Build history of the part. All positions in model axes, mm. A direction names the side the tool comes from. Give positions to 0.01 mm unless a question says otherwise; leave off trailing zeros. Loops run counter-clockwise (first coordinate to the right, second up) from the corner with the lowest first, then second, coordinate; pieces in that order, holes last. Notation, with made-up numbers: (64, 14) - (120, 14) arc R21 ccw to (120, 31) - close; hole circle Ø5 at (-3.75, 39.5). An arc over 180 degrees is marked (long way). Return JSON: item names as keys, results as strings. Group by question number.
1) Slice it at D-D (z = 1.25). List the corners of the cut face in (x, y).
2) Mould opens along X. For faces 1 (the face through (-53, -22, 3.48)), 2 (the face through (-45, -22, 3.48)), 3 (the face through (-50, -19, 0)), 4 (the face through (-41.453, -22, 2)) say: released by +X, released by -X, zero draft, split by the parting line, or undercut.
3) Slice it at A-A (z = 3). List the corners of the cut face in (x, y), and give its area (3 significant figures).
4) Drop a flat-ended pin along its axis: pin 1 (1.5 mm diameter, centred on x = -46, y = -22, fed in from -Z). Give the stop position or say it passes through.
5) Slice it at B-B (z = 4.3). List the corners of the cut face in (x, y), and give its area (3 significant figures).
6) Slice it at C-C (y = -20.25). List the corners of the cut face in (x, z) (3 decimals), and give its area (3 significant figures).
7) 3-axis set-ups, long thin cutter, end or side, ignore diameter. For faces 5 (the face through (-50, -25.879, 2)), 6 (the face through (-50, -22, 3.175)), 7 (the face through (-49, -24.279, 1)): which of +Z, -Z, +X, -X, +Y, -Y reach the whole face in a straight line?
8) Drill centre lines: probe 1 along X at (y, z) = (-23.5, 0.5); probe 2 along Y at (x, z) = (-49.5, 0.7); probe 3 along Z at (x, y) = (-53, -22.25). Where is each one in solid material? Low to high. Write a range as from..to.
```python
from build123d import *

# Parameters (mm, degrees)
F1_DEPTH = 3.175
F2_DEPTH = 5.08
F3_T     = -1.6002


with BuildPart() as f1:
    # F0 (on Top) → F1 (new body)
    with BuildSketch(Plane.XY):
        with BuildLine():
            Line((-53.3784843279, -17.9285755823), (-57.3535843279, -17.9285755823))
            Line((-57.3535843279, -17.9285755823), (-57.3535843279, -25.8787755823))
            Line((-57.3535843279, -25.8787755823), (-53.3784843279, -25.8787755823))
            Line((-53.3784843279, -25.8787755823), (-53.3784843279, -24.4436755823))
            ThreePointArc((-53.3784843279, -24.4436755823), (-55.9184843279, -21.9036755823), (-53.3784843279, -19.3636755823))
            Line((-53.3784843279, -19.3636755823), (-53.3784843279, -17.9285755823))
        make_face()
        with BuildLine():
            Line((-45.4282843279, -17.9285755823), (-53.3784843279, -17.9285755823))
            Line((-53.3784843279, -17.9285755823), (-53.3784843279, -19.3636755823))
            ThreePointArc((-53.3784843279, -19.3636755823), (-51.5824331037, -20.1076243581), (-50.8384843279, -21.9036755823))
            ThreePointArc((-50.8384843279, -21.9036755823), (-51.5824331037, -23.6997268065), (-53.3784843279, -24.4436755823))
            Line((-53.3784843279, -24.4436755823), (-53.3784843279, -25.8787755823))
            Line((-53.3784843279, -25.8787755823), (-45.4282843279, -25.8787755823))
            Line((-45.4282843279, -25.8787755823), (-45.4282843279, -24.4436755823))
            ThreePointArc((-45.4282843279, -24.4436755823), (-47.9682843279, -21.9036755823), (-45.4282843279, -19.3636755823))
            Line((-45.4282843279, -19.3636755823), (-45.4282843279, -17.9285755823))
        make_face()
        with BuildLine():
            Line((-41.4531843279, -17.9285755823), (-45.4282843279, -17.9285755823))
            Line((-45.4282843279, -17.9285755823), (-45.4282843279, -19.3636755823))
            ThreePointArc((-45.4282843279, -19.3636755823), (-43.6322331037, -20.1076243581), (-42.8882843279, -21.9036755823))
            ThreePointArc((-42.8882843279, -21.9036755823), (-43.6322331037, -23.6997268065), (-45.4282843279, -24.4436755823))
            Line((-45.4282843279, -24.4436755823), (-45.4282843279, -25.8787755823))
            Line((-45.4282843279, -25.8787755823), (-41.4531843279, -25.8787755823))
            Line((-41.4531843279, -25.8787755823), (-41.4531843279, -17.9285755823))
        make_face()
        with BuildLine():
            Line((-45.4282843279, -24.4436755823), (-45.4282843279, -19.3636755823))
            ThreePointArc((-45.4282843279, -19.3636755823), (-47.9682843279, -21.9036755823), (-45.4282843279, -24.4436755823))
        make_face()
        with BuildLine():
            ThreePointArc((-42.8882843279, -21.9036755823), (-43.6322331037, -20.1076243581), (-45.4282843279, -19.3636755823))
            Line((-45.4282843279, -19.3636755823), (-45.4282843279, -24.4436755823))
            ThreePointArc((-45.4282843279, -24.4436755823), (-43.6322331037, -23.6997268065), (-42.8882843279, -21.9036755823))
        make_face()
        with BuildLine():
            ThreePointArc((-50.8384843279, -21.9036755823), (-51.5824331037, -20.1076243581), (-53.3784843279, -19.3636755823))
            Line((-53.3784843279, -19.3636755823), (-53.3784843279, -24.4436755823))
            ThreePointArc((-53.3784843279, -24.4436755823), (-51.5824331037, -23.6997268065), (-50.8384843279, -21.9036755823))
        make_face()
        with BuildLine():
            Line((-53.3784843279, -24.4436755823), (-53.3784843279, -19.3636755823))
            ThreePointArc((-53.3784843279, -19.3636755823), (-55.9184843279, -21.9036755823), (-53.3784843279, -24.4436755823))
        make_face()
    extrude(amount=F1_DEPTH)

    # F0 (on Top) → F2 (join)
    with BuildSketch(Plane.XY):
        with BuildLine():
            Line((-53.3784843279, -24.4436755823), (-53.3784843279, -19.3636755823))
            ThreePointArc((-53.3784843279, -19.3636755823), (-55.9184843279, -21.9036755823), (-53.3784843279, -24.4436755823))
        make_face()
        with BuildLine():
            ThreePointArc((-50.8384843279, -21.9036755823), (-51.5824331037, -20.1076243581), (-53.3784843279, -19.3636755823))
            Line((-53.3784843279, -19.3636755823), (-53.3784843279, -24.4436755823))
            ThreePointArc((-53.3784843279, -24.4436755823), (-51.5824331037, -23.6997268065), (-50.8384843279, -21.9036755823))
        make_face()
        with BuildLine():
            Line((-45.4282843279, -24.4436755823), (-45.4282843279, -19.3636755823))
            ThreePointArc((-45.4282843279, -19.3636755823), (-47.9682843279, -21.9036755823), (-45.4282843279, -24.4436755823))
        make_face()
        with BuildLine():
            ThreePointArc((-42.8882843279, -21.9036755823), (-43.6322331037, -20.1076243581), (-45.4282843279, -19.3636755823))
            Line((-45.4282843279, -19.3636755823), (-45.4282843279, -24.4436755823))
            ThreePointArc((-45.4282843279, -24.4436755823), (-43.6322331037, -23.6997268065), (-42.8882843279, -21.9036755823))
        make_face()
    extrude(amount=F2_DEPTH)

    # F3
    f3_openings = [f1.faces().sort_by_distance(p)[0] for p in [
        (-49.403384, -21.903676, 0),
    ]]
    offset(amount=F3_T, openings=f3_openings, kind=Kind.INTERSECTION)


solid = f1.part
```
Results:
{
 "1": {"outline": "(-57.35, -25.88) - (-41.45, -25.88) - (-41.45, -17.93) - (-57.35, -17.93) - close; hole (-55.75, -24.28) - (-43.05, -24.28) - (-43.05, -19.53) - (-55.75, -19.53) - close"},
 "2": {"face 1": "undercut", "face 2": "undercut", "face 3": "zero draft", "face 4": "released by +X"},
 "3": {"outline": "(-57.35, -25.88) - (-41.45, -25.88) - (-41.45, -17.93) - (-57.35, -17.93) - close; hole circle Ø1.88 at (-53.38, -21.9); hole circle Ø1.88 at (-45.43, -21.9)", "area": "121 mm2"},
 "4": {"pin 1": "z = 1.57"},
 "5": {"outline": "circle Ø5.08 at (-53.38, -21.9); circle Ø5.08 at (-45.43, -21.9)", "area": "40.5 mm2"},
 "6": {"outline": "(-57.354, 0) - (-55.753, 0) - (-55.753, 1.575) - (-43.053, 1.575) - (-43.053, 0) - (-41.453, 0) - (-41.453, 3.175) - (-43.5, 3.175) - (-43.5, 5.08) - (-47.356, 5.08) - (-47.356, 3.175) - (-51.451, 3.175) - (-51.451, 5.08) - (-55.306, 5.08) - (-55.306, 3.175) - (-57.354, 3.175) - close", "area": "45.2 mm2"},
 "7": {"face 5": "+Z, -Z, +X, -X, -Y", "face 6": "+Z", "face 7": "-Z"},
 "8": {"probe 1": "-57.35..-55.75, -43.05..-41.45", "probe 2": "-25.88..-24.28, -19.53..-17.93", "probe 3": "3.48..5.08"}
}
